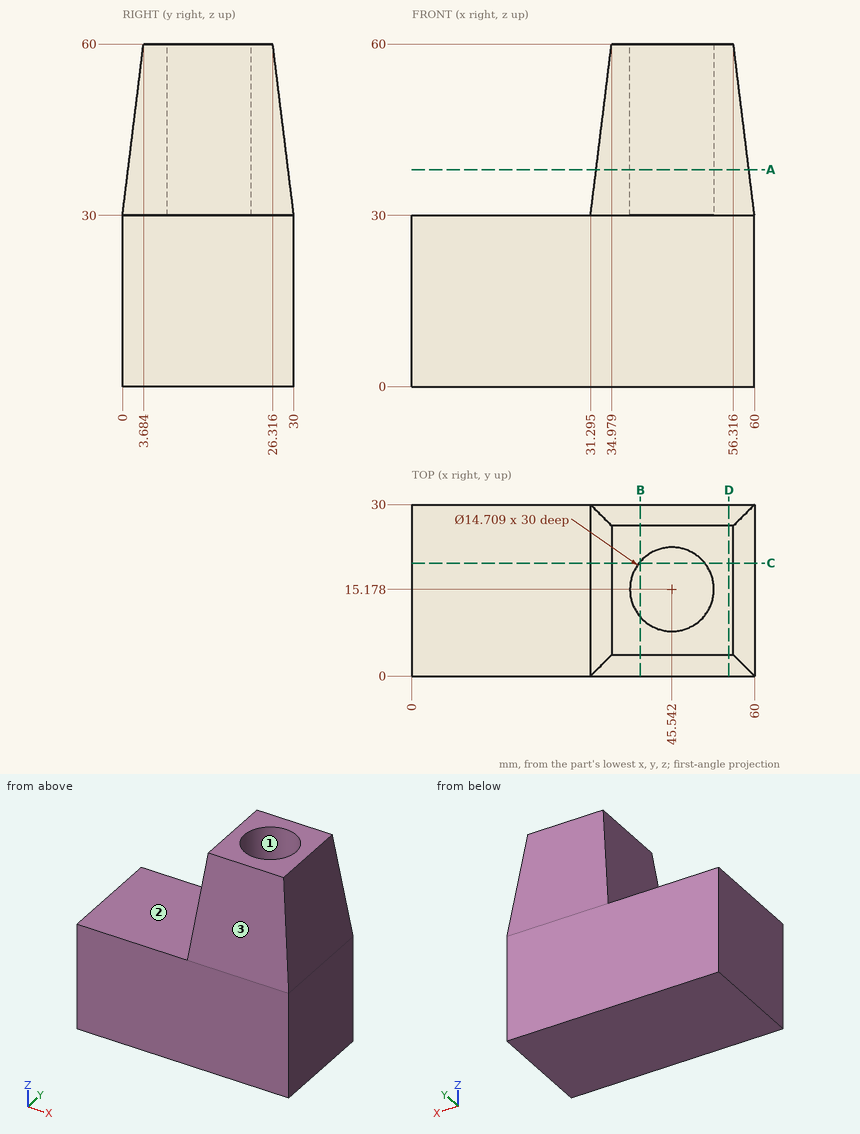
Check sheet for the drawn part. Datum: minimum x, y, z corner. Units: mm. Round coordinates to 2 decimals unless told otherwise and drop trailing zeros. Order: outer loops, then holes, each group sorted by start corner. A loop starts at its lowest first (then second) coordinate and runs counter-clockwise, first axis right, second up. Notation, with made-up numbers: M 20.25,57.5 L 34.25,57.5 A14 ccw 34.25,77.5 Z; hole C 4,66.25 d9. An arc over 180 degrees is marked long. Write each question's results on one line, items separated by ' | '. Start each with the question number.
1. Cross-section at A-A on z = 38. Record the boundary of the cut face in (x, y) (1 decimal).
2. Cross-section at D-D on x = 55.5. Record the boundary of the cut face in (y, z), plus the area to 3 significant figures.
3. Material ranges on L1, parallel to Z at x = 28.5, y = 5.25; L2, parallel to Y at x = 46, z = 38.5; L3, parallel to X at y = 16, z = 56, recorded low to high. Write a range as from..to.
4. Cross-section at C-C on y = 19.75. Record the boundary of the cut face in (x, z) (1 decimal), plus the area to 4 significant figures.
5. Go/stop test with flat-tipped pins: P1, Ø2, axis at x = 30, z = 9.5, coming from the -Y side; P2, Ø3, axis at x = 28.5, y = 5.5, coming from the +Z side. Record where each tip stops, or that it passes through.
6. Cross-section at B-B on x = 40. Record the boundary of the cut face in (y, z), plus the area to 3 significant figures.
7. Draft check along Y on the marked faces 1, 2 and 3. Enter one of: pulls with the +Y half, pulls with the -Y half, needs draft (parallel to the pull), parting line crosses it, or undercut.
Resolved:
1) outline: M 32.3,1 L 59,1 L 59,29 L 32.3,29 Z; hole C 45.5,15.2 d14.7
2) outline: M 0,0 L 30,0 L 30,30 L 26.32,60 L 3.68,60 L 0,30 Z | area: 1,690 mm2
3) L1: 0..30 | L2: 1.04..7.84, 22.52..28.96 | L3: 34.49..38.23, 52.85..56.81
4) outline: M 0,0 L 60,0 L 60,30 L 56.3,60 L 51.3,60 L 51.3,30 L 39.8,30 L 39.8,60 L 35,60 L 31.3,30 L 0,30 Z | area: 2,205 mm2
5) P1: y = 0 | P2: z = 30
6) outline: M 0,0 L 30,0 L 30,30 L 26.32,60 L 20.01,60 L 20.01,30 L 10.34,30 L 10.34,60 L 3.68,60 L 0,30 Z | area: 1,400 mm2
7) face 1: undercut | face 2: needs draft | face 3: pulls with the -Y half
